For this review, take the finished solid that the model builds, in its own axes (mm). A direction names the side the tool comes from. Round coordinates to 2 decimals unless told otherwise and drop trailing zeros. Write each loop counter-clockwise with the first axis right and the second up, starting at its lowest first coordinate (ties: lowest second). Pieces come first, ordered by that corner, then holes.
Autodesk Inventor part; units mm, degrees
ref_plane "YZ Plane" through (0, 0, 0) normal (1, 0, 0) x (0, 1, 0)
ref_plane "XZ Plane" through (0, 0, 0) normal (0, 1, 0) x (-1, 0, 0)
ref_plane "XY Plane" through (0, 0, 0) normal (0, 0, 1) x (1, 0, 0)
sketch "Sketch1" plane through (0, 0, 0) normal (0, 0, 1) x (1, 0, 0)
  circle A0 centre (0, 0) radius 361.95
  circle A1 centre (0, 0) radius 412.75
  dimension "d0" = 723.9
  dimension "d1" = 825.5
extrude "Extrusion1" add sketch "Sketch1" along normal blind 577
sketch "Sketch2" plane through (0, 0, 0) normal (0, 0, -1) x (-1, 0, 0)
  circle A0 centre (0, 0) radius 412.75
  circle A1 centre (0, 0) radius 415.925
  dimension "d4" = 831.85
extrude "Extrusion2" add sketch "Sketch2" against normal blind 50.8
sketch "Sketch3" plane through (0, 0, 0) normal (0, 0, -1) x (-1, 0, 0)
  circle A0 centre (0, 0) radius 415.925
  circle A1 centre (0, 0) radius 412.496
  dimension "d7" = 824.992
extrude "Extrusion3" cut sketch "Sketch3" against normal blind 25.4
chamfer "Chamfer1" distance 3.175 angle 45 1 edges at (-412.75, 0, 50.8)
sketch "Sketch4" plane through (0, 0, 577) normal (0, 0, 1) x (1, 0, 0)
  circle A0 centre (0, 0) radius 361.95
  circle A1 centre (0, 0) radius 387.096
  dimension "d13" = 774.192
extrude "Extrusion4" add sketch "Sketch4" along normal blind 12.7
fillet "Fillet1" radius 0.7937 2 edges at (-387.096, 0, 577) (412.496, 0, 25.4)
chamfer "Chamfer2" distance 0.7937 angle 45 1 edges at (-387.096, 0, 589.7)
equation "\"d10\" = -0.5 * d1 + 0.5 * d4"
properties part number "A1-19027-100-06 HCWI liner - pup" material "Iron, HCWI"
(1) For line 1 along Y through (x, z) = (0, 252); line 2 along X through (y, z) = (218, 172.5); line 3 along X through (y, z) = (296.5, 484), list the stretches that pass through material, from the lowest coordinate up.
Geometry check:
line 1: y = -412.75 to -361.95, 361.95 to 412.75
line 2: x = -350.48 to -288.94, 288.94 to 350.48
line 3: x = -287.14 to -207.59, 207.59 to 287.14
(2) For pin 1 Ø12 at (y, z) = (127, 199) entering from -X; pin 2 Ø4 at (y, z) = (0, 319) entering from -X; pin 3 Ø8 at (x, z) = (-159.5, 158) entering from -Y; pin 4 Ø12 at (x, y) = (146, -327.5) entering from +Z, all flat-tipped, find the tip position at first contact; note any pin that passes through.
Geometry check:
pin 1: stops at x = -394.62
pin 2: stops at x = -412.75
pin 3: stops at y = -382.34
pin 4: stops at z = 589.7
(3) We need section C-C, the plane z = 415.5. Give the boundary of the cut face in (x, y).
Geometry check:
outline: circle Ø825.5 at (0, 0); hole circle Ø723.9 at (0, 0)
(4) Mouldability with a two-part tool opening along Y and no side actions: class faces 4 (the face through (2, -365, 0)), 5 (the face through (-47.12, -358.87, 290.72)), 6 (the face through (-327.544, 251.152, 311.826)) as pulls with the +Y half, pulls with the -Y half, needs draft (parallel to the pull), parting line crosses it, or undercut.
Geometry check:
face 4: needs draft
face 5: undercut
face 6: parting line crosses it
(5) For faces 1 (the face through (53.699, 408.986, 12.131)), 2 (the face through (113, 345, 589.7)), 3 (the face through (-50.4, -383.8, 583.3)), list the 3-axis set-ups (+Z, -Z, +X, -X, +Y, -Y) from which the entire face can be reached by the end or side of a thin tool; tool diameter is ignored.
Geometry check:
face 1: -Z
face 2: +Z, +X, -X, +Y, -Y
face 3: +Z
